Work out the finished part from the listing and answer in its coordinate system (mm). A direction names the side the tool comes from. Round coordinates to 2 decimals unless told otherwise and drop trailing zeros. Order: outer loops, then holes, each group sorted by start corner. A loop starts at its lowest first (then second) coordinate and runs counter-clockwise, first axis right, second up. Notation, with made-up numbers: (31.5, -9.75) - (44.5, -9.75) arc R33 cw to (44.5, 29.25) - close; hole circle Ø6 at (6, 0.5). An arc over 180 degrees is marked (long way). Use one line per item in the form item = value. Start each with the question number.
Q1. Which of the six approach directions +Z, -Z, +X, -X, +Y, -Y give full straight-line access (tool end or side, diameter ignored) to faces 4 (the cylindrical face through (-0.011, -0.913, 4.586)), 5 (the flat face through (2, -0.6, 0)), 6 (the flat face through (-2, -1.2, 0))?
Q2. The part is cut by section D-D on z = -3. Determine the outline of the cut face in (x, y), plus the area to 3 significant figures.
Q3. The part is cut by section C-C on y = -1.55. Determine the outline of the cut face in (x, z), plus the area to 3 significant figures.
Q4. Given P1, Ø3, axis at x = -2.5, z = -1.5, coming from the -Y side; P2, Ø1, axis at x = 0.5, y = -1, coming from the +Z side; P3, Ø3, axis at x = 3.5, z = -1, coming from the +Y side, each flat-ended and moving along its own axis, determine where each tip first touches the part or whether it passes through.
Q5. The part is cut by section A-A on z = 0. Determine the outline of the cut face in (x, y), plus the area to 3 significant figures.
Q6. Find the intervals of material crossed by line 1 (Z direction, x = 0, y = -1.4); line 2 (X direction, y = -0.65, z = 0); line 3 (X direction, y = -0.25, z = 3), in increasing order. Write a range as [from, to].
Q7. The part is cut by section B-B on x = 0. Determine the outline of the cut face in (y, z), plus the area to 3 significant figures.
Q8. For a pull along X with two mould halves and no side action, classify faces 1 (the cylindrical face through (-0.065, -0.913, -2.504)), 2 (the flat face through (1, -1.8, 0)), 3 (the flat face through (-2, -1, 3)) as +X half, -X half, draft (parallel to the pull), parting line (faces both ways), or undercut.
from build123d import *

# Parameters (mm, degrees)
F1_DEPTH = 1.8
F2_DEPTH = 1.2
F4_DEPTH = 0.6
F5_R     = 1
F6_R     = 0.5
F7_DEPTH = 12.5


with BuildPart() as f1:
    # F0 (on Front) → F1 (new body)
    with BuildSketch(Plane.XZ):
        with BuildLine():
            Line((5, 0), (0, 5))
            Line((0, 5), (-1.249147, 3.750853))
            ThreePointArc((-1.249147, 3.750853), (-0.864917, 0), (-1.249147, -3.750853))
            Line((-1.249147, -3.750853), (0, -5))
            Line((0, -5), (5, 0))
        make_face()
    extrude(amount=F1_DEPTH)

    # F0 (on Front) → F2 (join)
    with BuildSketch(Plane.XZ):
        with BuildLine():
            ThreePointArc((-1.249147, -3.750853), (-0.864917, 0), (-1.249147, 3.750853))
            Line((-1.249147, 3.750853), (-5, 0))
            Line((-5, 0), (-1.249147, -3.750853))
        make_face()
    extrude(amount=F2_DEPTH)

    # F3 (on face) → F4 (cut)
    with BuildSketch(Plane.XZ):
        with BuildLine():
            ThreePointArc((1.249147, 3.750853), (0.864917, 0), (1.249147, -3.750853))
            Line((1.249147, -3.750853), (5, 0))
            Line((5, 0), (1.249147, 3.750853))
        make_face()
    extrude(amount=F4_DEPTH, mode=Mode.SUBTRACT)

    # F5
    f5_edges = [f1.edges().sort_by_distance(p)[0] for p in [
        (0, -0.9, 5),
        (5, -1.2, 0),
        (0, -0.9, -5),
        (-5, -0.6, 0),
    ]]
    fillet(f5_edges, radius=F5_R)

    # F6 (on Front) → F7 (cut, symmetric)
    with BuildSketch(Plane.XZ):
        with Locations((-2.725786, 0)):
            Circle(F6_R)
        with Locations((2.725786, 0)):
            Circle(F6_R)
        with Locations((0, 3)):
            Circle(F6_R)
        with Locations((0, -3)):
            Circle(F6_R)
    extrude(amount=F7_DEPTH, both=True, mode=Mode.SUBTRACT)


solid = f1.part
Found:
q1.face_4 = +Z, +Y, -Y
q1.face_5 = +X, +Y
q1.face_6 = -X, -Y
q2.outline = (-2, -1.2) - (-1.11, -1.2) - (-1.11, -1.8) - (-0.5, -1.8) - (-0.5, 0) - (-2, 0) - close; (0.5, -1.8) - (2, -1.8) - (2, -0.6) - (1.11, -0.6) - (1.11, 0) - (0.5, 0) - close
q2.area = 4.33 mm²
q3.outline = (-1.25, -3.75) - (-0.71, -4.29) arc R1 ccw to (0.71, -4.29) - (4.29, -0.71) arc R1 ccw to (4.29, 0.71) - (0.71, 4.29) arc R1 ccw to (-0.71, 4.29) - (-1.25, 3.75) arc R18.5 cw to start; hole circle Ø1 at (0, -3); hole circle Ø1 at (0, 3); hole circle Ø1 at (2.73, 0)
q3.area = 31.0 mm²
q4.P1 = -1.2
q4.P2 = 4.59
q4.P3 = -0.6
q5.outline = (-4.59, -1.2) - (-3.23, -1.2) - (-3.23, 0) - (-4.59, 0) - close; (-2.23, -1.2) - (-0.86, -1.2) - (-0.86, -1.8) - (2.23, -1.8) - (2.23, -0.6) - (0.86, -0.6) - (0.86, 0) - (-2.23, 0) - close; (3.23, -1.8) - (4.59, -1.8) - (4.59, -0.6) - (3.23, -0.6) - close
q5.area = 9.64 mm²
q6.line_1 = [-4.59, -3.5], [-2.5, 2.5], [3.5, 4.59]
q6.line_2 = [-4.59, -3.23], [-2.23, 2.23], [3.23, 4.59]
q6.line_3 = [-2, -0.5], [0.5, 1.11]
q7.outline = (-1.8, -4.59) - (0, -4.59) - (0, -3.5) - (-1.8, -3.5) - close; (-1.8, -2.5) - (0, -2.5) - (0, 2.5) - (-1.8, 2.5) - close; (-1.8, 3.5) - (0, 3.5) - (0, 4.59) - (-1.8, 4.59) - close
q7.area = 12.9 mm²
q8.face_1 = undercut
q8.face_2 = draft
q8.face_3 = -X half
